The model under review builds one solid part; all positions refer to its coordinate system, in mm. Give positions to 0.01 mm unless a question says otherwise; leave off trailing zeros. Loops run counter-clockwise (first coordinate to the right, second up) from the corner with the lowest first, then second, coordinate; pieces in that order, holes last. Notation, with made-up numbers: M 41,26.25 L 90,26.25 A18 ccw 90,55.25 Z; hole C 74.5,1.5 d1. An arc over 180 degrees is marked long. Return JSON: item names as keys, results as strings.
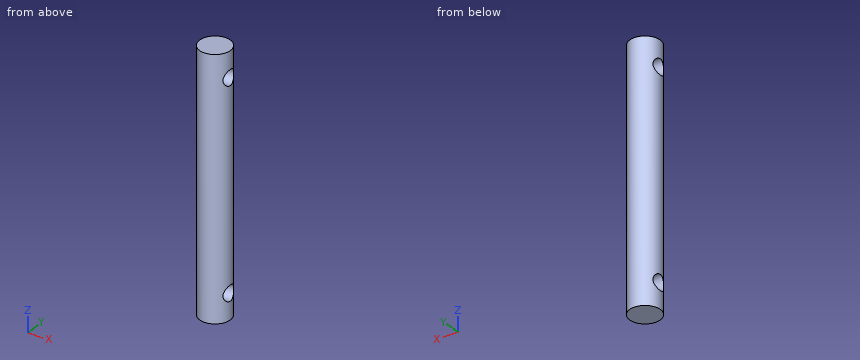
```python
from build123d import *

# Parameters (mm, degrees)
SKETCH1_R               = 3
BOSS_EXTRUDE1_DEPTH     = 50
SKETCH2_R               = 1.5
CUT_EXTRUDE1_DEPTH      = 4
CUT_EXTRUDE1_DEPTH_BACK = 4


with BuildPart() as part:
    # Sketch1 → Boss-Extrude1 (new body)
    with BuildSketch(Plane.XY):
        Circle(SKETCH1_R)
    extrude(amount=BOSS_EXTRUDE1_DEPTH)

    # Sketch2 → Cut-Extrude1 (cut, two sides)
    with BuildSketch(Plane(origin=(0, 0, 0), x_dir=(0, 0, -1), z_dir=(1, 0, 0))) as cut_extrude1_sk:
        with Locations((-45, 0)):
            Circle(SKETCH2_R)
        with Locations((-5, 0)):
            Circle(SKETCH2_R)
    extrude(amount=CUT_EXTRUDE1_DEPTH, mode=Mode.SUBTRACT)
    extrude(cut_extrude1_sk.sketch, amount=-CUT_EXTRUDE1_DEPTH_BACK, mode=Mode.SUBTRACT)


solid = part.part
```
1) Consider section D-D on y = -2. Write out the cut boundary in (x, z), then the cut area to 3 significant figures.
From the geometry:
{"outline": "M -2.24,0 L 2.24,0 L 2.24,50 L -2.24,50 Z", "area": "224 mm²"}
2) Wall thickness on L1, parallel to Z at x = -1.1, y = 0; L2, parallel to Z at x = -2, y = -0.5; L3, parallel to Y at x = 1.85, z = 45: over which ranges is each line inside the solid? List them lowest first. Write a range as from..to.
From the geometry:
{"L1": "0..3.5, 6.5..43.5, 46.5..50", "L2": "0..3.59, 6.41..43.59, 46.41..50", "L3": "-2.36..-1.5, 1.5..2.36"}
3) Consider section B-B on z = 5. Write out the cut boundary in (x, y).
From the geometry:
{"outline": "M -2.6,-1.5 A3 ccw 2.6,-1.5 Z; M -2.6,1.5 L 2.6,1.5 A3 ccw Z"}
4) Consider section A-A on y = 0. Write out the cut boundary in (x, z).
From the geometry:
{"outline": "M -3,0 L 3,0 L 3,3.5 L -3,3.5 Z; M -3,6.5 L 3,6.5 L 3,43.5 L -3,43.5 Z; M -3,46.5 L 3,46.5 L 3,50 L -3,50 Z"}
5) Insertion check: pin 1 (3 mm diameter, centred on x = 2, z = 36, fed in from -Y); pin 2 (3.5 mm diameter, centred on y = 0, z = 5, fed in from -X); pin 3 (3 mm diameter, centred on x = 2.5, z = 19.5, fed in from -Y); pin 4 (1 mm diameter, centred on y = -1.5, z = 41.5, fed in from -X). Each pin has a flat end and moves straight along its axis. Give the tip position at first contact, or say it passes through.
From the geometry:
{"pin 1": "y = -2.96", "pin 2": "x = -3", "pin 3": "y = -2.83", "pin 4": "x = -2.83"}
6) Consider section C-C on x = -0.75. Write out the cut boundary in (y, z).
From the geometry:
{"outline": "M -2.9,0 L 2.9,0 L 2.9,50 L -2.9,50 Z; hole C 0,5 d3; hole C 0,45 d3"}
